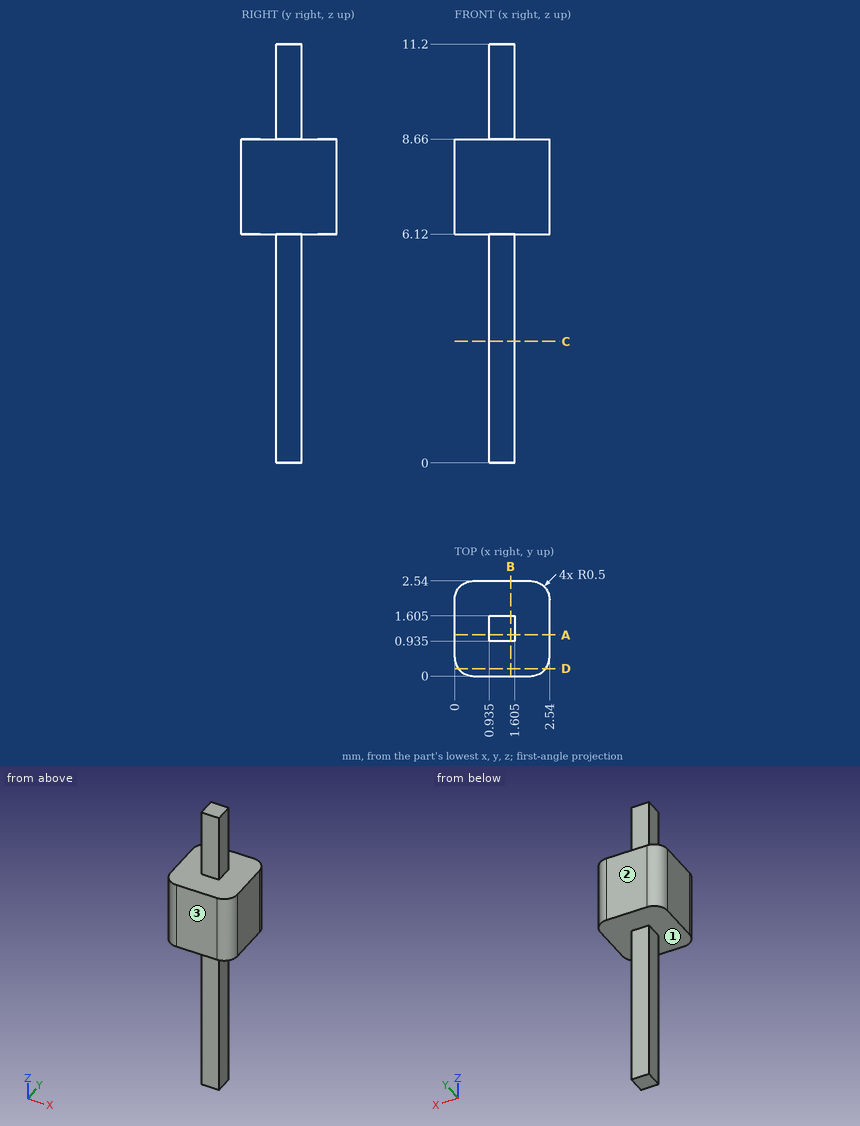
Input: dimensioned drawing with shaded views. Units: mm. Origin: part minimum x, y, z. Give positions to 0.01 mm unless a question says otherwise; leave off trailing zeros. Write each loop counter-clockwise with the first axis right and the second up, starting at its lowest first coordinate (ties: lowest second). Pieces come first, ordered by that corner, then holes. Notation, with made-up numbers: (59, 74) -> (63, 74) arc R19 ccw to (63, 103) -> close; hole circle Ø3 at (-9, 69). An arc over 180 degrees is marked (long way). Return JSON: item names as keys, results as strings. Group by question number.
1. Section A-A, the plane y = 1.1. Output: boundary loops of the cut face in (x, z) (3 decimals).
2. Section C-C, the plane z = 3.25. Output: boundary loops of the cut face in (x, y) (3 decimals).
3. Mould query, pull axis Y, two halves, no side actions, for the marked faces 1, 2 and 3. Classes: +Y half, -Y half, draft (parallel to the pull), parting line (faces both ways), or undercut.
4. Section D-D, the plane y = 0.2. Output: boundary loops of the cut face in (x, z), then the cut area to 3 significant figures.
5. Pin query (flat end, axial travel): pin 1 Ø1 at (x, y) = (0.5, 1) entering from +Z; pin 2 Ø0.5 at (x, z) = (1.5, 9.5) entering from +Y (3 decimals); pin 3 Ø0.7 at (y, z) = (1.5, 10) entering from -X (3 decimals); pin 4 Ø0.7 at (y, z) = (1.5, 2.5) entering from +X (3 decimals). Return the tip coordinate at first contact, or that it passes through.
6. Material intervals for line 1 (Z direction, x = 1.3, y = 1.95); line 2 (X direction, y = 1.5, z = 0.75) (3 decimals), sorted ascending. Write a range as from..to.
Determined:
{
 "1": {"outline": "(0, 6.12) -> (0.935, 6.12) -> (0.935, 0) -> (1.605, 0) -> (1.605, 6.12) -> (2.54, 6.12) -> (2.54, 8.66) -> (1.605, 8.66) -> (1.605, 11.2) -> (0.935, 11.2) -> (0.935, 8.66) -> (0, 8.66) -> close"},
 "2": {"outline": "(0.935, 0.935) -> (1.605, 0.935) -> (1.605, 1.605) -> (0.935, 1.605) -> close"},
 "3": {"face 1": "draft", "face 2": "+Y half", "face 3": "-Y half"},
 "4": {"outline": "(0.1, 6.12) -> (2.44, 6.12) -> (2.44, 8.66) -> (0.1, 8.66) -> close", "area": "5.94 mm2"},
 "5": {"pin 1": "stops at z = 11.2", "pin 2": "stops at y = 1.605", "pin 3": "stops at x = 0.935", "pin 4": "stops at x = 1.605"},
 "6": {"line 1": "z = 6.12..8.66", "line 2": "x = 0.935..1.605"}
}
